For this review, take the finished solid that the model builds, in its own axes (mm). Round coordinates to 2 decimals unless told otherwise and drop trailing zeros. Order: outer loops, then holes, each group sorted by start corner. A loop starts at its lowest first (then second) coordinate and runs counter-clockwise, first axis right, second up. Notation, with made-up numbers: (-10.75, -36) - (7.25, -36) arc R24 cw to (7.25, -25) - close; hole circle Ø3 at (51.25, -31). An arc over 180 degrees is marked (long way). Write each question's results on one line, items separated by ' | '. Start each with the question number.
(1) For L1, parallel to Y at x = 16, z = 1.25; L2, parallel to X at y = -33, z = 2.5; L3, parallel to X at y = -6.5, z = 9.5, list the stretches that pass through material, from the lowest coordinate up. Write a range as from..to.
(2) Insertion check: pin 1 Ø5 at (x, z) = (67, 4) entering from -Y; pin 2 Ø3 at (x, y) = (-5.5, -53) entering from -Z; pin 3 Ø1 at (x, z) = (-6, 6) entering from +Y; pin 4 Ø2.5 at (y, z) = (-57, 1) entering from -X. Each pin has a flat end and moves straight along its axis. Give the tip position at first contact, or say it passes through.
(3) Take a section at B-B, the plane x = 68.5. Give the boundary of the cut face in (y, z), plus the area to 3 significant figures.
(4) Take a section at A-A, the plane y = -41. Give the boundary of the cut face in (x, z).
(5) Take a section at C-C, the plane y = -97.5. Give the boundary of the cut face in (x, z).
(6) Take a section at D-D, the plane z = 1.5. Give the boundary of the cut face in (x, y), plus the area to 3 significant figures.
```python
from build123d import *

# Parameters (mm, degrees)
F0_W      = 2
F0_H      = 3
F1_DEPTH  = 100
F2_W      = 78
F2_H      = 90
F1_FACE_W = 6
F1_FACE_H = 100
F3_DEPTH  = 3
F4_W      = 6
F4_H      = 12
F5_DEPTH  = 10
F7_D      = 4
F7_DEPTH  = 8.001
F9_D      = 4


# Not quite as in the source:
# - a feature names something its author has since deleted; it is built from what else it names


with BuildPart() as f1:
    # F0 (on Front) → F1 (new body)
    with BuildSketch(Plane.XZ):
        Polygon((-2, 0), (0, 0), (86, 0), (86, 10), (84, 10), (84, 3), (0, 3), (0, 7), (-2, 7), (-8, 7), (-8, 5), (-2, 5), align=None)
        with Locations((-1, 8.5)):
            Rectangle(F0_W, F0_H)
    extrude(amount=F1_DEPTH)

    # F2 (on Top) + F1_face (on face) → F3 (cut)
    with BuildSketch(Plane.XY):
        with Locations((42, -50)):
            Rectangle(F2_W, F2_H)
    with BuildSketch(Plane(origin=(-5, -50, 7), x_dir=(1, 0, 0), z_dir=(0, 0, 1))):
        Rectangle(F1_FACE_W, F1_FACE_H)
    extrude(amount=F3_DEPTH, mode=Mode.SUBTRACT)

    # F4 (on Top) → F5 (cut)
    with BuildSketch(Plane.XY):
        with Locations((-5, -6)):
            Rectangle(F4_W, F4_H)
    extrude(amount=F5_DEPTH, mode=Mode.SUBTRACT)

    # F7 (through all, one way)
    with BuildSketch(Plane.YZ):
        with Locations((-2.5, 7.5), (-97.5, 7.5)):
            Circle(F7_D / 2)
    extrude(amount=-F7_DEPTH, mode=Mode.SUBTRACT)

    # F9 (through all)
    with Locations(Plane(origin=(0, 0, 0), x_dir=(0, 1, 0), z_dir=(-1, 0, 0))):
        with Locations((-2.5, -7.5), (-97.5, -7.5)):
            Hole(F9_D / 2)


solid = f1.part
```
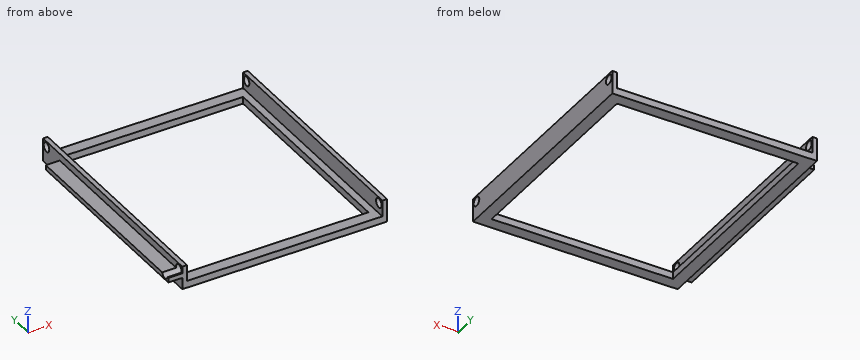
Results below:
1) L1: y = -100..-95, -5..0 | L2: x = -2..3, 81..86 | L3: x = -2..0, 84..86
2) pin 1: stops at y = -100 | pin 2: stops at z = 5 | pin 3: stops at y = -12 | pin 4: stops at x = -2
3) outline: (-100, 0) - (-95, 0) - (-95, 3) - (-100, 3) - close; (-5, 0) - (0, 0) - (0, 3) - (-5, 3) - close | area: 30.0 mm^2
4) outline: (-8, 5) - (-2, 5) - (-2, 0) - (3, 0) - (3, 3) - (0, 3) - (0, 10) - (-2, 10) - (-2, 7) - (-8, 7) - close; (81, 0) - (86, 0) - (86, 10) - (84, 10) - (84, 3) - (81, 3) - close
5) outline: (-8, 5) - (-2, 5) - (-2, 0) - (86, 0) - (86, 5.5) - (84, 5.5) - (84, 3) - (0, 3) - (0, 5.5) - (-8, 5.5) - close; (-2, 9.5) - (0, 9.5) - (0, 10) - (-2, 10) - close; (84, 9.5) - (86, 9.5) - (86, 10) - (84, 10) - close
6) outline: (-2, -100) - (86, -100) - (86, 0) - (-2, 0) - close; hole (3, -95) - (81, -95) - (81, -5) - (3, -5) - close | area: 1,780 mm^2
